```python
from build123d import *

# Parameters (mm, degrees)
SKETCH1_W           = 18.6
SKETCH1_H           = 26.2
SKETCH1_R           = 1.25
BOSS_EXTRUDE1_DEPTH = 1.2
SKETCH3_W           = 12.2
SKETCH3_H           = 12
BOSS_EXTRUDE2_DEPTH = 4.4
SKETCH10_W          = 1.45
SKETCH10_H          = 0.2
SKETCH13_W          = 1.45
SKETCH13_H          = 0.2
LPATTERN1_COUNT     = 2
LPATTERN1_PITCH     = 2.85
LPATTERN2_COUNT     = 2
LPATTERN2_PITCH     = 2.85
SKETCH14_R          = 3.5
BOSS_EXTRUDE4_DEPTH = 7.1
CHAMFER1_SIZE       = 0.3
SKETCH15_R          = 1.9
BOSS_EXTRUDE5_DEPTH = 0.65
SKETCH16_R          = 3
BOSS_EXTRUDE6_DEPTH = 14.45
CHAMFER2_SIZE       = 0.6
CUT_EXTRUDE1_DEPTH  = 10.8
SKETCH18_R          = 0.35
CUT_EXTRUDE2_DEPTH  = 1.2
SKETCH19_W          = 1.5
SKETCH19_H          = 2.5
SKETCH19_R          = 0.35
BOSS_EXTRUDE7_DEPTH = 0.01
FILLET1_R           = 0.5


with BuildPart() as part:
    # Sketch1 → Boss-Extrude1 (new body)
    with BuildSketch(Plane(origin=(0, 0, 0), x_dir=(1, 0, 0), z_dir=(0, 1, 0))):
        Rectangle(SKETCH1_W, SKETCH1_H)
        with Locations((-7.3, 8.3)):
            Circle(SKETCH1_R, mode=Mode.SUBTRACT)
        with Locations((-7.3, -5.4)):
            Circle(SKETCH1_R, mode=Mode.SUBTRACT)
    extrude(amount=BOSS_EXTRUDE1_DEPTH)

    # Sketch3 → Boss-Extrude2 (add)
    with BuildSketch(Plane(origin=(0, 1.2, 0), x_dir=(1, 0, 0), z_dir=(0, 1, 0))):
        with Locations((1.1, 2.8)):
            Rectangle(SKETCH3_W, SKETCH3_H)
    extrude(amount=BOSS_EXTRUDE2_DEPTH)

    # Sweep3: sweep along a curve in space
    with BuildLine() as sweep3_path:
        Line((-1.325, 2.85, 3.2), (-1.325, 2.85, 4.3))
        ThreePointArc((-1.325, 2.85, 4.3), (-1.325, 2.703553391, 4.653553391), (-1.325, 2.35, 4.8))
        Line((-1.325, 2.35, 4.8), (-1.325, 1.2, 4.8))
    # Sketch10 → Sweep3 (sweep)
    with BuildSketch(Plane.XY.offset(3.2)):
        with Locations((-1.325, 2.85)):
            Rectangle(SKETCH10_W, SKETCH10_H)
    sweep3 = sweep(path=sweep3_path.line)

    # Mirror2: Sweep3 across plane
    add(sweep3.mirror(Plane.ZY.offset(-1.1)))

    # Sweep4: sweep along a curve in space
    with BuildLine() as sweep4_path:
        Line((1.1, 2.8, -8.8), (1.1, 2.8, -9.75))
        ThreePointArc((1.1, 2.8, -9.75), (1.1, 2.653553391, -10.103553391), (1.1, 2.3, -10.25))
        Line((1.1, 2.3, -10.25), (1.1, 1.2, -10.25))
    # Sketch13 → Sweep4 (sweep)
    with BuildSketch(Plane(origin=(0, 0, -8.8), x_dir=(-1, 0, 0), z_dir=(0, 0, -1))):
        with Locations((-1.1, 2.8)):
            Rectangle(SKETCH13_W, SKETCH13_H)
    sweep4 = sweep(path=sweep4_path.line)

    # LPattern1: Sweep4 ×2
    with Locations(*[(-i * LPATTERN1_PITCH, 0, 0) for i in range(1, LPATTERN1_COUNT)]):
        add(sweep4)

    # LPattern2: Sweep4 ×2
    with Locations(*[(i * LPATTERN2_PITCH, 0, 0) for i in range(1, LPATTERN2_COUNT)]):
        add(sweep4)

    # Sketch14 → Boss-Extrude4 (add)
    with BuildSketch(Plane(origin=(0, 5.6, 0), x_dir=(1, 0, 0), z_dir=(0, 1, 0))):
        with Locations((1.1, 2.8)):
            Circle(SKETCH14_R)
    extrude(amount=BOSS_EXTRUDE4_DEPTH)

    # Chamfer1
    chamfer1_edges = [part.edges().sort_by_distance(p)[0] for p in [
        (-2.4, 12.7, -2.8),
    ]]
    chamfer(chamfer1_edges, length=CHAMFER1_SIZE)

    # Sketch15 → Boss-Extrude5 (add)
    with BuildSketch(Plane(origin=(0, 12.7, 0), x_dir=(1, 0, 0), z_dir=(0, 1, 0))):
        with Locations((1.1, 2.8)):
            Circle(SKETCH15_R)
    extrude(amount=BOSS_EXTRUDE5_DEPTH)

    # Sketch16 → Boss-Extrude6 (add)
    with BuildSketch(Plane(origin=(0, 13.35, 0), x_dir=(1, 0, 0), z_dir=(0, 1, 0))):
        with Locations((1.1, 2.8)):
            Circle(SKETCH16_R)
    extrude(amount=BOSS_EXTRUDE6_DEPTH)

    # Chamfer2
    chamfer2_edges = [part.edges().sort_by_distance(p)[0] for p in [
        (-1.9, 27.8, -2.8),
    ]]
    chamfer(chamfer2_edges, length=CHAMFER2_SIZE)

    # Sketch17 → Cut-Extrude1 (cut)
    with BuildSketch(Plane(origin=(0, 27.8, 0), x_dir=(1, 0, 0), z_dir=(0, 1, 0))):
        with BuildLine():
            Line((-0.396662955, 5.4), (-0.396662955, 0.2))
            ThreePointArc((-0.396662955, 0.2), (-1.9, 2.8), (-0.396662955, 5.4))
        make_face()
    extrude(amount=-CUT_EXTRUDE1_DEPTH, mode=Mode.SUBTRACT)

    # Sketch18 → Cut-Extrude2 (cut)
    with BuildSketch(Plane(origin=(0, 1.2, 0), x_dir=(1, 0, 0), z_dir=(0, 1, 0))):
        with Locations((6.5, -11)):
            Circle(SKETCH18_R)
        with Locations((3.96, -11)):
            Circle(SKETCH18_R)
        with Locations((1.42, -11)):
            Circle(SKETCH18_R)
        with Locations((-1.12, -11)):
            Circle(SKETCH18_R)
        with Locations((-3.66, -11)):
            Circle(SKETCH18_R)
    extrude(amount=-CUT_EXTRUDE2_DEPTH, mode=Mode.SUBTRACT)

    # Sketch19 → Boss-Extrude7 (add)
    with BuildSketch(Plane(origin=(0, 1.2, 0), x_dir=(1, 0, 0), z_dir=(0, 1, 0))):
        with Locations((3.96, -11)):
            Rectangle(SKETCH19_W, SKETCH19_H)
        with Locations((3.96, -11)):
            Circle(SKETCH19_R, mode=Mode.SUBTRACT)
        with Locations((6.5, -11)):
            Rectangle(SKETCH19_W, SKETCH19_H)
        with Locations((6.5, -11)):
            Circle(SKETCH19_R, mode=Mode.SUBTRACT)
        with Locations((1.42, -11)):
            Rectangle(SKETCH19_W, SKETCH19_H)
        with Locations((1.42, -11)):
            Circle(SKETCH19_R, mode=Mode.SUBTRACT)
        with Locations((-1.12, -11)):
            Rectangle(SKETCH19_W, SKETCH19_H)
        with Locations((-1.12, -11)):
            Circle(SKETCH19_R, mode=Mode.SUBTRACT)
        with Locations((-3.66, -11)):
            Rectangle(SKETCH19_W, SKETCH19_H)
        with Locations((-3.66, -11)):
            Circle(SKETCH19_R, mode=Mode.SUBTRACT)
    boss_extrude7 = extrude(amount=BOSS_EXTRUDE7_DEPTH)

    # Mirror3: Boss-Extrude7 across plane
    add(boss_extrude7.mirror(Plane.ZX.offset(0.6)))

    # Fillet1
    fillet1_edges = [part.edges().sort_by_distance(p)[0] for p in [
        (7.2, 3.4, 3.2),
        (7.2, 3.4, -8.8),
        (-5, 3.4, -8.8),
        (-5, 3.4, 3.2),
    ]]
    fillet(fillet1_edges, radius=FILLET1_R)


solid = part.part
```
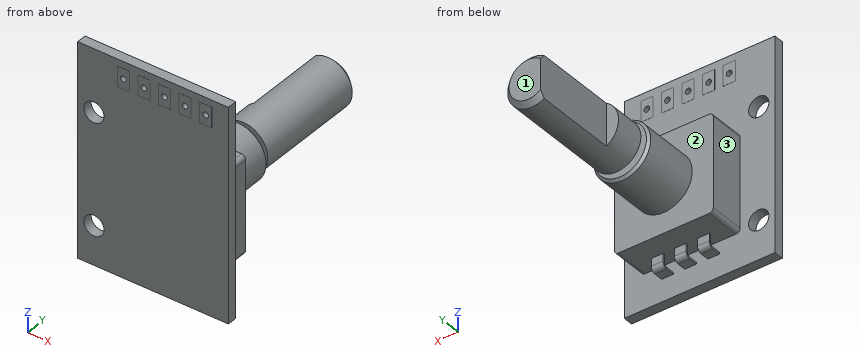
Geometry: final body of the model. Coordinates: model frame, mm. Face numbers are marked on the shaded views. A direction names the side the tool comes from. Round coordinates to 2 decimals unless told otherwise and drop trailing zeros. Order: outer loops, then holes, each group sorted by start corner. A loop starts at its lowest first (then second) coordinate and runs counter-clockwise, first axis right, second up. Notation, with made-up numbers: (10, -23) -> (36, -23) arc R16 ccw to (36, -15) -> close; hole circle Ø5 at (11.25, -35). An arc over 180 degrees is marked (long way). Use one line per item in the form item = value. Start each with the question number.
1. Line query: probe 1 along X at (y, z) = (0.95, 11); probe 2 along Z at (x, y) = (-7.3, 0.45); probe 3 along Z at (x, y) = (6.5, 0.5). Output: solid intervals per line, ascending.
2. Reachability of the marked faces 1, 2 and 3 from +Z, -Z, +X, -X, +Y, -Y: full face, straight path, thin tool, end or side. Return the list, or none.
3. Cut plane C-C (x = -7.3). Return the cut outline in (y, z).
4. Cut plane B-B (z = 3.75). Return the cut outline in (x, y).
5. Pin query (flat end, axial travel): pin 1 Ø10 at (y, z) = (14.5, 6) entering from -X; pin 2 Ø0.5 at (x, z) = (4.5, -9) entering from -Y; pin 3 Ø6 at (x, y) = (5, 6) entering from +Z; pin 4 Ø3.5 at (x, y) = (0.5, 4) entering from -Z. Return the tip coordinate at first contact, or that it passes through.
6. Cut plane D-D (z = -2.8). Return the cut outline in (x, y).
Solution:
q1.probe_1 = -9.3 to -4.01, -3.31 to -1.47, -0.77 to 1.07, 1.77 to 3.61, 4.31 to 6.15, 6.85 to 9.3
q1.probe_2 = -13.1 to -9.55, -7.05 to 4.15, 6.65 to 13.1
q1.probe_3 = -13.1 to 10.65, 11.35 to 13.1
q2.face_1 = +Z, -Z, +X, -X, +Y
q2.face_2 = +Y
q2.face_3 = +Z, -Z, -X, +Y
q3.outline = (0, -13.1) -> (1.2, -13.1) -> (1.2, -9.55) -> (0, -9.55) -> close; (0, -7.05) -> (1.2, -7.05) -> (1.2, 4.15) -> (0, 4.15) -> close; (0, 6.65) -> (1.2, 6.65) -> (1.2, 13.1) -> (0, 13.1) -> close
q4.outline = (-9.3, 0) -> (9.3, 0) -> (9.3, 1.2) -> (-9.3, 1.2) -> close; (-2.05, 2.75) -> (-0.6, 2.75) -> (-0.6, 2.95) -> (-2.05, 2.95) -> close; (2.8, 2.75) -> (4.25, 2.75) -> (4.25, 2.95) -> (2.8, 2.95) -> close
q5.pin_1 = through
q5.pin_2 = 0
q5.pin_3 = 3.2
q5.pin_4 = -10.35
q6.outline = (-9.3, 0) -> (9.3, 0) -> (9.3, 1.2) -> (7.2, 1.2) -> (7.2, 5.6) -> (4.6, 5.6) -> (4.6, 12.4) -> (4.3, 12.7) -> (3, 12.7) -> (3, 13.35) -> (4.1, 13.35) -> (4.1, 27.2) -> (3.5, 27.8) -> (-0.4, 27.8) -> (-0.4, 17) -> (-1.9, 17) -> (-1.9, 13.35) -> (-0.8, 13.35) -> (-0.8, 12.7) -> (-2.1, 12.7) -> (-2.4, 12.4) -> (-2.4, 5.6) -> (-5, 5.6) -> (-5, 1.2) -> (-9.3, 1.2) -> close
